For this review, take the finished solid that the model builds, in its own axes (mm). A direction names the side the tool comes from. Coordinates: 2 decimals unless noted, no trailing zeros. Loops run counter-clockwise (first coordinate to the right, second up) from the corner with the lowest first, then second, coordinate; pieces in that order, holes last. Notation, with made-up numbers: (-17.5, 26.5) -> (25.5, 26.5) arc R16 cw to (25.5, 55.5) -> close; hole circle Ø6 at (32.25, 51.5). An arc over 180 degrees is marked (long way). Answer in a Markdown table with one row per item.
Autodesk Inventor part; units mm, degrees
ref_plane "YZ Plane" through (0, 0, 0) normal (1, 0, 0) x (0, 1, 0)
ref_plane "XZ Plane" through (0, 0, 0) normal (0, 1, 0) x (-1, 0, 0)
ref_plane "XY Plane" through (0, 0, 0) normal (0, 0, 1) x (1, 0, 0)
sketch "Sketch1" plane through (0, 0, 0) normal (0, 1, 0) x (-1, 0, 0)
  line L0 (0, 3.2563) -> (2.82, 1.6281)
  line L1 (2.82, 1.6281) -> (2.82, -1.6281)
  line L2 (2.82, -1.6281) -> (0, -3.2563)
  line L3 (0, -3.2563) -> (-2.82, -1.6281)
  line L4 (-2.82, -1.6281) -> (-2.82, 1.6281)
  line L5 (-2.82, 1.6281) -> (0, 3.2563)
  point P0 (0, 0)
  point P1 (0, 0)
  dimension "d0" = 5.64
extrude "Extrusion1" add sketch "Sketch1" along normal blind 18
sketch "Sketch2" plane through (0, 18, 0) normal (0, 1, 0) x (1, 0, 0)
  point P0 (0, 0)
  point P1 (0, 0)
hole "Hole1" at (0, 18, 0) direction (0, -1, 0) diameter 2.013 depth 7.6 tip angle 118 countersink diameter 4.5 countersink angle 82
sketch "Sketch3" plane through (0, 0, 0) normal (0, -1, 0) x (1, 0, 0)
  circle A0 centre (0, 0) radius 1.25
  dimension "d10" = 2.5
extrude "Extrusion2" add sketch "Sketch3" along normal blind 5.75
thread "Thread1"
chamfer "Chamfer1" distance 0.5 angle 45 1 edges at (-1.25, -5.75, 0)
properties part number "2.5x18mm Standoff" material "Bronze, Soft Tin"
Item 1: Take a section at A-A, the plane y = 16.25. State the section outline as (x, z) points, and give its area (3 significant figures).
Worked answers:
| item | result |
|---|---|
| outline | (-2.82, -1.63) -> (0, -3.26) -> (2.82, -1.63) -> (2.82, 1.63) -> (0, 3.26) -> (-2.82, 1.63) -> close; hole circle Ø2.01 at (0, 0) |
| area | 24.4 mm² |
Item 2: The part is to be moulded in two halves that separate along Z. For faces 4 (the conical face through (0.05, 9.9, 0.17)), 5 (the cylindrical face through (-0.27, -2.59, 1.22)), 6 (the flat face through (2.82, 9, 0)), 7 (the flat face through (-1.39, 8.874, 2.454)), say which applies: +Z half, -Z half, draft (parallel to the pull), parting line (faces both ways), or undercut.
Worked answers:
| item | result |
|---|---|
| face 4 | undercut |
| face 5 | parting line |
| face 6 | draft |
| face 7 | +Z half |
Item 3: Take a section at B-B, the plane y = -1.25. State the section outline as (x, z) points.
Worked answers:
| item | result |
|---|---|
| outline | circle Ø2.5 at (0, 0) |
Item 4: For faces 1 (the flat face through (0, -5.75, 0)), 2 (the cylindrical face through (0.983, 13.442, -0.218)), 3 (the flat face through (0.04, 0, -1.4)), list the 3-axis set-ups (+Z, -Z, +X, -X, +Y, -Y) from which the entire face can be reached by the end or side of a thin tool; tool diameter is ignored.
Worked answers:
| item | result |
|---|---|
| face 1 | +Z, -Z, +X, -X, -Y |
| face 2 | +Y |
| face 3 | -Y |
Item 5: Insertion check: pin 1 (1.2 mm diameter, centred on x = 0, z = 0, fed in from +Y); pin 2 (1.5 mm diameter, centred on x = -2, y = 0.5, fed in from +Z); pin 3 (1.5 mm diameter, centred on x = 1, z = 0, fed in from +Y). Each pin has a flat end and moves straight along its axis. Give the tip position at first contact, or say it passes through.
Worked answers:
| item | result |
|---|---|
| pin 1 | y = 10.16 |
| pin 2 | z = 2.53 |
| pin 3 | y = 17.42 |
Item 6: Take a section at C-C, the plane y = 6.5. State the section outline as (x, z) points, and give its area (3 significant figures).
Worked answers:
| item | result |
|---|---|
| outline | (-2.82, -1.63) -> (0, -3.26) -> (2.82, -1.63) -> (2.82, 1.63) -> (0, 3.26) -> (-2.82, 1.63) -> close |
| area | 27.5 mm² |
Item 7: For L1, parallel to X at y = 14.25, z = 0; L2, parallel to Y at x = -1.65, z = -1.75; L3, parallel to X at y = 15.75, z = 0.5, list the stretches that pass through material, from the lowest coordinate up.
Worked answers:
| item | result |
|---|---|
| L1 | -2.82 to -1.01, 1.01 to 2.82 |
| L2 | 0 to 18 |
| L3 | -2.82 to -0.87, 0.87 to 2.82 |
